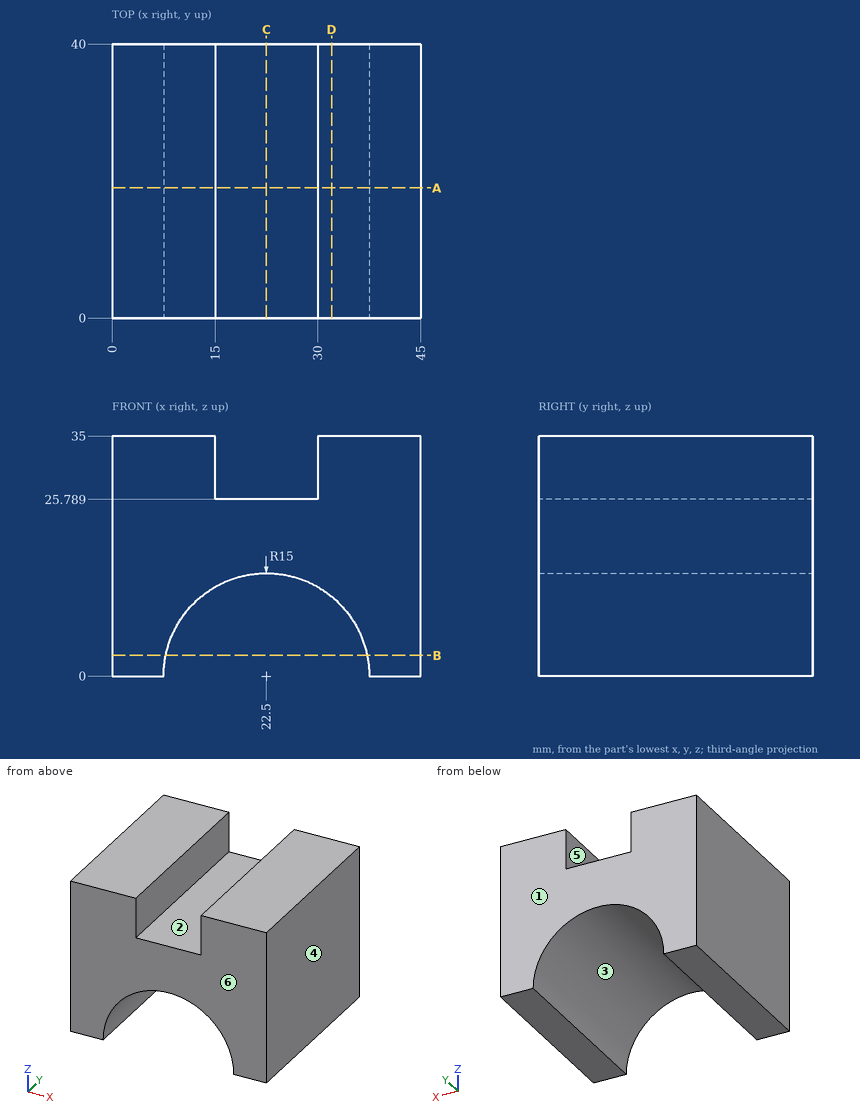
For this review, use the dimensioned drawing (mm, ordinates from the lowest corner) and the shaded views. A direction names the side the tool comes from. Round coordinates to 2 decimals unless told otherwise and drop trailing zeros. Order: outer loops, then holes, each group sorted by start corner. A loop starts at its lowest first (then second) coordinate and runs counter-clockwise, first axis right, second up. Notation, with made-up numbers: (40.25, 81) -> (60.25, 81) arc R27 ccw to (60.25, 112) -> close; hole circle Ø8 at (69.5, 38.5). An arc over 180 degrees is marked (long way). Write item = value, one per line. Start each with the question number.
Item 1: Consider section C-C on x = 22.5. Write out the cut boundary in (y, z).
Item 2: Consider section B-B on z = 3. Write out the cut boundary in (x, y), plus the area to 3 significant figures.
Item 3: For the marked faces 1 and 2, list the 3-axis set-ups (+Z, -Z, +X, -X, +Y, -Y) from which the entire face can be reached by the end or side of a thin tool; tool diameter is ignored.
Item 4: For line 1 along X through (y, z) = (11, 31); line 2 along X through (y, z) = (33, 4.5); line 3 along Z through (x, y) = (34, 14.5), list the stretches that pass through material, from the lowest coordinate up.
Item 5: Mouldability with a two-part tool opening along X and no side actions: class the marked faces 3, 4, 5 and 6 as released by +X, released by -X, zero draft, split by the parting line, or undercut.
Item 6: Consider section A-A on y = 19. Write out the cut boundary in (x, z), plus the area to 3 significant figures.
Item 7: Clearance check with flat-ended pins moving along their axes: pin 1 Ø1 at (x, y) = (25, 35) entering from -Z; pin 2 Ø12 at (x, y) = (23, 19) entering from +Z; pin 3 Ø1 at (x, z) = (19, 27) entering from +Y (3 decimals); pin 4 Ø5 at (x, y) = (16.5, 26.5) entering from -Z. State where each tip first meets the part, or that it passes through.
Item 8: Consider section D-D on x = 32. Write out the cut boundary in (y, z), plus the area to 3 significant figures.
Conclusion:
q1.outline = (0, 15) -> (40, 15) -> (40, 25.79) -> (0, 25.79) -> close
q2.outline = (0, 0) -> (7.8, 0) -> (7.8, 40) -> (0, 40) -> close; (37.2, 0) -> (45, 0) -> (45, 40) -> (37.2, 40) -> close
q2.area = 624 mm2
q3.face_1 = +Z, -Z, +X, -X, +Y
q3.face_2 = +Z, +Y, -Y
q4.line_1 = 0 to 15, 30 to 45
q4.line_2 = 0 to 8.19, 36.81 to 45
q4.line_3 = 9.63 to 35
q5.face_3 = undercut
q5.face_4 = released by +X
q5.face_5 = undercut
q5.face_6 = zero draft
q6.outline = (0, 0) -> (7.5, 0) arc R15 cw to (37.5, 0) -> (45, 0) -> (45, 35) -> (30, 35) -> (30, 25.79) -> (15, 25.79) -> (15, 35) -> (0, 35) -> close
q6.area = 1,080 mm2
q7.pin_1 = 14.7
q7.pin_2 = 25.79
q7.pin_3 = through
q7.pin_4 = 12.36
q8.outline = (0, 11.61) -> (40, 11.61) -> (40, 35) -> (0, 35) -> close
q8.area = 936 mm2
